from build123d import *

# Parameters (mm, degrees)
F0_W     = 104.0384
F0_H     = 22.4536
F1_DEPTH = 1.651
F2_R     = 1.9
F3_DEPTH = 6.35
F4_R     = 1.5875
F5_R     = 1.397
F6_DEPTH = 1.651
F7_W     = 21.717
F7_H     = 8.382
F8_DEPTH = 4.445


with BuildPart() as f1:
    # F0 (on Front) → F1 (new body)
    with BuildSketch(Plane.XZ):
        with Locations((52.0192, 11.2268)):
            Rectangle(F0_W, F0_H)
    extrude(amount=F1_DEPTH)

    # F2 (on face) → F3 (join)
    with BuildSketch(Plane.XZ.offset(1.651)):
        with Locations((20.32, 5.842)):
            Circle(F2_R)
    extrude(amount=F3_DEPTH)

    # F4
    f4_edges = [f1.edges().sort_by_distance(p)[0] for p in [
        (18.42, -8.001, 5.842),
    ]]
    fillet(f4_edges, radius=F4_R)

    # F5 (on face) → F6 (cut, through all)
    with BuildSketch(Plane.XZ.offset(1.651)):
        with Locations((10.033, 14.4526)):
            Circle(F5_R)
        with Locations((94.7674, 14.4526)):
            Circle(F5_R)
    extrude(amount=-F6_DEPTH, mode=Mode.SUBTRACT)

    # F7 (on face) → F8 (join)
    with BuildSketch(Plane.XZ.offset(1.651)):
        with Locations((52.0192, 20.6756)):
            Rectangle(F7_W, F7_H)
    extrude(amount=F8_DEPTH)


solid = f1.part
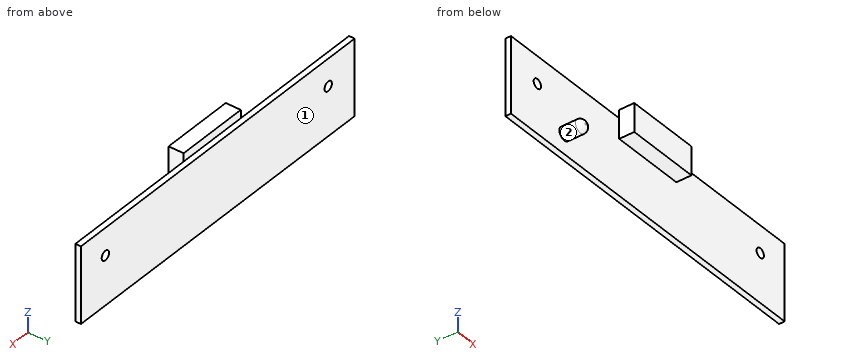
Work out the finished part from the listing and answer in its coordinate system (mm). Face numbers are marked on the shaded views. A direction names the side the tool comes from. Coordinates: 2 decimals unless noted, no trailing zeros. Write each loop counter-clockwise with the first axis right and the second up, starting at its lowest first coordinate (ties: lowest second). Pieces come first, ordered by that corner, then holes. Notation, with made-up numbers: (41, 43) - (97, 43) arc R20 cw to (97, 76) - close; hole circle Ø1 at (72.25, 75). An arc over 180 degrees is marked (long way). One line per question, with ' | ' between items.
1) Consider probe 1 along Y at (x, z) = (79.5, 10.5); probe 2 along X at (y, z) = (-5.5, 22.25); probe 3 along Z at (x, y) = (15, -0.25). Determine where each line is inside the solid, lowest interval first. Write a range as [from, to].
Checks:
probe 1: [-1.65, 0] | probe 2: [41.16, 62.88] | probe 3: [0, 22.45]
2) Find section B-B, the plane x = 59. Determine the outline of the cut face in (y, z).
Checks:
outline: (-6.1, 16.48) - (-1.65, 16.48) - (-1.65, 0) - (0, 0) - (0, 22.45) - (-1.65, 22.45) - (-1.65, 24.87) - (-6.1, 24.87) - close
3) Find section A-A, the plane z = 20. Determine the outline of the cut face in (x, y).
Checks:
outline: (0, -1.65) - (41.16, -1.65) - (41.16, -6.1) - (62.88, -6.1) - (62.88, -1.65) - (104.04, -1.65) - (104.04, 0) - (0, 0) - close
4) Flat-ended cylindrical pins translate along their axes: P1, Ø3, axis at x = 60, z = 3, coming from the +Y side; P2, Ø4, axis at x = 41.5, z = 8, coming from the -Y side; P3, Ø1.8, axis at x = 68.5, y = -1, coming from the +Z side; P4, Ø1.3, axis at x = 49.5, y = -3, coming from the -Z side. Find the tip coordinate at first contact, or state that the pin passes through.
Checks:
P1: y = 0 | P2: y = -1.65 | P3: z = 22.45 | P4: z = 16.48
5) For the marked faces 1 and 2, determine the directions among +Z, -Z, +X, -X, +Y, -Y from which every point of the face is accessible in a straight line to the end or side of a thin tool.
Checks:
face 1: +Z, -Z, +X, -X, +Y | face 2: -Y
6) Find section C-C, the plane x = 12.5. Determine the outline of the cut face in (y, z).
Checks:
outline: (-1.65, 0) - (0, 0) - (0, 22.45) - (-1.65, 22.45) - close
